Geometry check sheet. Reference: the model listing, model coordinates, mm. Face numbers are marked on the shaded views. Give positions to 0.01 mm unless a question says otherwise; leave off trailing zeros. Order: outer loops, then holes, each group sorted by start corner. A loop starts at its lowest first (then second) coordinate and runs counter-clockwise, first axis right, second up.
```python
from build123d import *

# Parameters (mm, degrees)
SKETCH1_R           = 22.5
BOSS_EXTRUDE1_DEPTH = 12.7
SKETCH2_R           = 3.3
CUT_EXTRUDE1_DEPTH  = 35.260618792


with BuildPart() as part:
    # Sketch1 → Boss-Extrude1 (new body)
    with BuildSketch(Plane(origin=(0, 0, 0), x_dir=(1, 0, 0), z_dir=(0, 1, 0))):
        with Locations(Location((0, 0, 0), (0, 0, 270))):
            Circle(SKETCH1_R)
    extrude(amount=BOSS_EXTRUDE1_DEPTH)

    # Sketch2 → Cut-Extrude1 (cut, through all)
    with BuildSketch(Plane(origin=(0, 12.7, 0), x_dir=(1, 0, 0), z_dir=(0, 1, 0))):
        with Locations(Location((-16, 0, 0), (0, 0, 270))):
            Circle(SKETCH2_R)
        with Locations(Location((-11.313708499, 11.313708499, 0), (0, 0, 270))):
            Circle(SKETCH2_R)
        with Locations(Location((0, 16, 0), (0, 0, 270))):
            Circle(SKETCH2_R)
        with Locations(Location((11.313708499, 11.313708499, 0), (0, 0, 270))):
            Circle(SKETCH2_R)
        with Locations(Location((16, 0, 0), (0, 0, 270))):
            Circle(SKETCH2_R)
        with Locations(Location((11.313708499, -11.313708499, 0), (0, 0, 270))):
            Circle(SKETCH2_R)
        with Locations(Location((0, -16, 0), (0, 0, 270))):
            Circle(SKETCH2_R)
        with Locations(Location((-11.313708499, -11.313708499, 0), (0, 0, 270))):
            Circle(SKETCH2_R)
    extrude(amount=-CUT_EXTRUDE1_DEPTH, mode=Mode.SUBTRACT)


solid = part.part
```
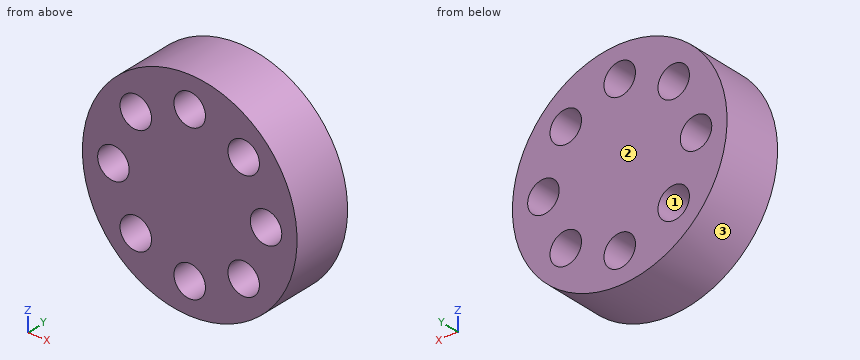
Q1. Cross-section at C-C, the plane x = -13.5. Record the boundary of the cut face in (y, z), and give its area (3 significant figures).
Q2. Gauge pin test, flat ends, axial feed: P1, Ø6, axis at x = 0, z = -16, coming from the -Y side; P2, Ø3, axis at x = -8.5, y = 10, coming from the -Z side; P3, Ø1, axis at x = -9, y = 9, coming from the -Z side; P4, Ø1.5, axis at y = 4.5, z = 9, coming from the -X side. Record the tip position at first contact, or that the pin passes through.
Q3. Thickness scan on L1, parallel to X at y = 5.25, z = 0; L2, parallel to Z at x = 11.5, y = 10.75; L3, parallel to Z at x = -0.5, y = 2.25. Record the ranges inside material, lowest first.
Q4. Release check for a two-part mould opening along X. For the marked faces 1, 2 and 3 record: pulls with the +X half, pulls with the -X half, needs draft (parallel to the pull), parting line crosses it, or undercut.
Q5. Cross-section at D-D, the plane z = -15.5. Record the boundary of the cut face in (x, y), and give its area (3 significant figures).
Q6. Cross-section at A-A, the plane x = 0. Record the boundary of the cut face in (y, z).
Q7. Cross-section at B-B, the plane z = 0. Record the boundary of the cut face in (x, y).
Answers follow:
1. outline: (0, -18) - (12.7, -18) - (12.7, -13.79) - (0, -13.79) - close; (0, -8.84) - (12.7, -8.84) - (12.7, -2.15) - (0, -2.15) - close; (0, 2.15) - (12.7, 2.15) - (12.7, 8.84) - (0, 8.84) - close; (0, 13.79) - (12.7, 13.79) - (12.7, 18) - (0, 18) - close
1. area: 277 mm2
2. P1: passes through
2. P2: stops at z = -21.38
2. P3: stops at z = -20.83
2. P4: stops at x = -20.93
3. L1: x = -22.5 to -19.3, -12.7 to 12.7, 19.3 to 22.5
3. L2: z = -19.34 to -14.61, -8.02 to 8.02, 14.61 to 19.34
3. L3: z = -22.49 to -19.26, -12.74 to 12.74, 19.26 to 22.49
4. face 1: undercut
4. face 2: needs draft
4. face 3: parting line crosses it
5. outline: (-16.31, 0) - (-3.26, 0) - (-3.26, 12.7) - (-16.31, 12.7) - close; (3.26, 0) - (16.31, 0) - (16.31, 12.7) - (3.26, 12.7) - close
5. area: 331 mm2
6. outline: (0, -22.5) - (12.7, -22.5) - (12.7, -19.3) - (0, -19.3) - close; (0, -12.7) - (12.7, -12.7) - (12.7, 12.7) - (0, 12.7) - close; (0, 19.3) - (12.7, 19.3) - (12.7, 22.5) - (0, 22.5) - close
7. outline: (-22.5, 0) - (-19.3, 0) - (-19.3, 12.7) - (-22.5, 12.7) - close; (-12.7, 0) - (12.7, 0) - (12.7, 12.7) - (-12.7, 12.7) - close; (19.3, 0) - (22.5, 0) - (22.5, 12.7) - (19.3, 12.7) - close
